Verification items for the finished model (mm, model axes). Face numbers are marked on the shaded views. A direction names the side the tool comes from. Coordinates: 2 decimals unless noted, no trailing zeros. Order: outer loops, then holes, each group sorted by start corner. A loop starts at its lowest first (then second) coordinate and runs counter-clockwise, first axis right, second up. Notation, with made-up numbers: (45.25, 10.5) - (72.25, 10.5) arc R27 ccw to (72.25, 43.5) - close; hole circle Ø8 at (-30, 28). An arc over 180 degrees is marked (long way). Answer as CSV lines item,"result". Start each with the question number.
1. Mould release check, pull along X, two halves, no side actions. Record for the marked faces 3, 4, 5 and 6: pulls with the +X half, pulls with the -X half, needs draft (parallel to the pull), parting line crosses it, or undercut.
2. Set-up check for the marked faces 1 and 2: record each of +Z, -Z, +X, -X, +Y, -Y from which the full face is reachable in a straight line by a thin tool's end or side.
3. Section check D-D (z = -77). Record the cut outline in (x, y).
4. Section check B-B (y = 68). Record the cut outline in (x, z), and give its area (3 significant figures).
5. Material ranges on L1, parallel to X at y = 29, z = -83; L2, parallel to Z at x = 27, y = 14.5; L3, parallel to X at y = 78, z = 28, recorded low to high. Write a range as [from, to].
6. Go/stop test with flat-tipped pins: pin 1 (4 mm diameter, centred on y = 106.5, z = -67, fed in from -X); pin 2 (12 mm diameter, centred on x = 65, y = 70, fed in from -Z); pin 3 (1 mm diameter, centred on x = -100, y = 103, fed in from +Z); pin 4 (4 mm diameter, centred on x = -110, y = 54.5, fed in from +Z). Record where each tip stops, or that it passes through.
7. Section check A-A (z = 5.5). Record the cut outline in (x, y), and give its area (3 significant figures).
8. Section check C-C (x = -56.5). Record the cut outline in (y, z).
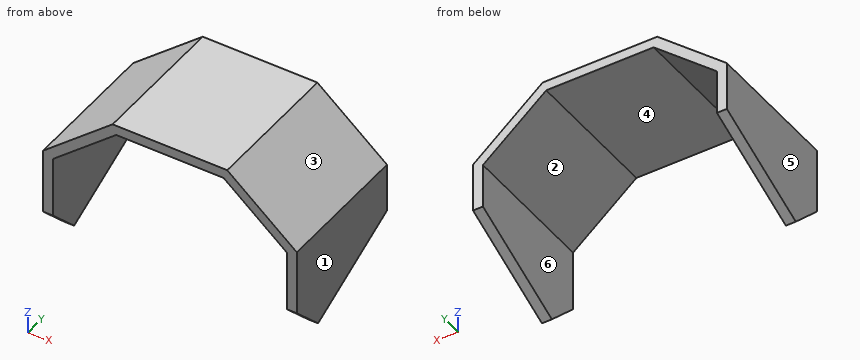
from build123d import *

# Parameters (mm, degrees)
F1_DEPTH = 170
F3_DEPTH = 350
F5_DEPTH = 400


with BuildPart() as f1:
    # F0 (on Front) → F1 (new body)
    with BuildSketch(Plane.XZ):
        Polygon((-141.604444, 18.745599), (-65, 83.02436), (65, 83.02436), (141.604444, 18.745599), (141.604444, -95.024361), (153.604444, -95.024361), (153.604444, 24.341291), (69.367643, 95.02436), (-69.367643, 95.02436), (-153.604444, 24.341291), (-153.604444, -95.024361), (-141.604444, -95.024361), align=None)
    extrude(amount=-F1_DEPTH)

    # F2 (on face) → F3 (cut)
    with BuildSketch(Plane.YZ.offset(153.604444)):
        Polygon((170, -35.341535), (40, -95.024361), (170, -95.024361), align=None)
    extrude(amount=-F3_DEPTH, mode=Mode.SUBTRACT)

    # F4 (on face) → F5 (cut)
    with BuildSketch(Plane.YZ.offset(153.604444)):
        Polygon((0, -95.024361), (40, -95.024361), (0, -55.024361), align=None)
    extrude(amount=-F5_DEPTH, mode=Mode.SUBTRACT)


solid = f1.part
Evaluation:
1,face 3,"pulls with the +X half"
1,face 4,"undercut"
1,face 5,"pulls with the -X half"
1,face 6,"undercut"
2,face 1,"+Z, -Z, +X, +Y, -Y"
2,face 2,"-Z, +Y, -Y"
3,outline,"(-153.6, 21.98) - (-141.6, 21.98) - (-141.6, 79.26) - (-153.6, 79.26) - close; (141.6, 21.98) - (153.6, 21.98) - (153.6, 79.26) - (141.6, 79.26) - close"
4,outline,"(-153.6, -82.17) - (-141.6, -82.17) - (-141.6, 18.75) - (-65, 83.02) - (65, 83.02) - (141.6, 18.75) - (141.6, -82.17) - (153.6, -82.17) - (153.6, 24.34) - (69.37, 95.02) - (-69.37, 95.02) - (-153.6, 24.34) - close"
4,area,"6,620 mm²"
5,L1,"x = [-153.6, -141.6], [141.6, 153.6]"
5,L2,"z = [83.02, 95.02]"
5,L3,"x = [-149.24, -130.58], [130.58, 149.24]"
6,pin 1,"passes through"
6,pin 2,"stops at z = 77.99"
6,pin 3,"stops at z = 69.74"
6,pin 4,"stops at z = 62.61"
7,outline,"(-153.6, 0) - (-141.6, 0) - (-141.6, 170) - (-153.6, 170) - close; (141.6, 0) - (153.6, 0) - (153.6, 170) - (141.6, 170) - close"
7,area,"4,080 mm²"
8,outline,"(0, 83.02) - (170, 83.02) - (170, 95.02) - (0, 95.02) - close"
